Check sheet for the modelled part. Datum: model origin and axes. Units: mm. Face numbers are marked on the shaded views. Coordinates: 2 decimals unless noted, no trailing zeros. Loops run counter-clockwise (first coordinate to the right, second up) from the corner with the lowest first, then second, coordinate; pieces in that order, holes last.
```python
from build123d import *

# Parameters (mm, degrees)
SKETCH013_W     = 47
SKETCH013_H     = 14.8
PAD005_DEPTH    = 3
SKETCH014_R     = 0.95
POCKET003_DEPTH = 5
SKETCH015_R     = 0.95
POCKET004_DEPTH = 2
SKETCH016_W     = 40
SKETCH016_H     = 12.6
PAD006_DEPTH    = 1.5
SKETCH017_R     = 2.5
POCKET005_DEPTH = 10
CHAMFER014_SIZE = 0.5
CHAMFER015_SIZE = 0.5
CHAMFER016_SIZE = 0.2


with BuildPart() as part:
    # Sketch013 → Pad005 (new body)
    with BuildSketch(Plane.YZ):
        with Locations((0, 4.5)):
            Rectangle(SKETCH013_W, SKETCH013_H)
    extrude(amount=PAD005_DEPTH)

    # Sketch014 → Pocket003 (cut)
    with BuildSketch(Plane.YZ):
        with Locations((-21.7, 4.5)):
            Circle(SKETCH014_R)
        with Locations((21.7, 4.5)):
            Circle(SKETCH014_R)
    extrude(amount=POCKET003_DEPTH, mode=Mode.SUBTRACT)

    # Sketch015 → Pocket004 (cut)
    with BuildSketch(Plane.YZ.offset(3)):
        with Locations((-21.7, 4.5)):
            Circle(SKETCH015_R)
        with Locations((21.7, 4.5)):
            Circle(SKETCH015_R)
    extrude(amount=-POCKET004_DEPTH, mode=Mode.SUBTRACT)

    # Sketch016 → Pad006 (join)
    with BuildSketch(Plane.YZ):
        with Locations((0, 4.5)):
            Rectangle(SKETCH016_W, SKETCH016_H)
    extrude(amount=-PAD006_DEPTH)

    # Sketch017 → Pocket005 (cut)
    with BuildSketch(Plane(origin=(3, 15, 4.5), x_dir=(0, 1, 0), z_dir=(1, 0, 0))):
        Circle(SKETCH017_R)
    extrude(amount=-POCKET005_DEPTH, mode=Mode.SUBTRACT)

    # Chamfer014
    chamfer014_edges = [part.edges().sort_by_distance(p)[0] for p in [
        (-1.5, 12.5, 4.5),
        (3, 12.5, 4.5),
    ]]
    chamfer(chamfer014_edges, length=CHAMFER014_SIZE)

    # Chamfer015
    chamfer015_edges = [part.edges().sort_by_distance(p)[0] for p in [
        (-1.5, 20, 4.5),
        (-1.5, 0, -1.8),
        (-1.5, -20, 4.5),
        (-1.5, 0, 10.8),
    ]]
    chamfer(chamfer015_edges, length=CHAMFER015_SIZE)

    # Chamfer016
    chamfer016_edges = [part.edges().sort_by_distance(p)[0] for p in [
        (0, 23.5, 4.5),
        (0, 0, -2.9),
        (0, 0, 11.9),
        (0, -23.5, 4.5),
    ]]
    chamfer(chamfer016_edges, length=CHAMFER016_SIZE)


with BuildPart() as part_1:
    # Body003 placement: moved
    add(part.part.moved(Location((22, 0, 5))))


solid = part_1.part
```
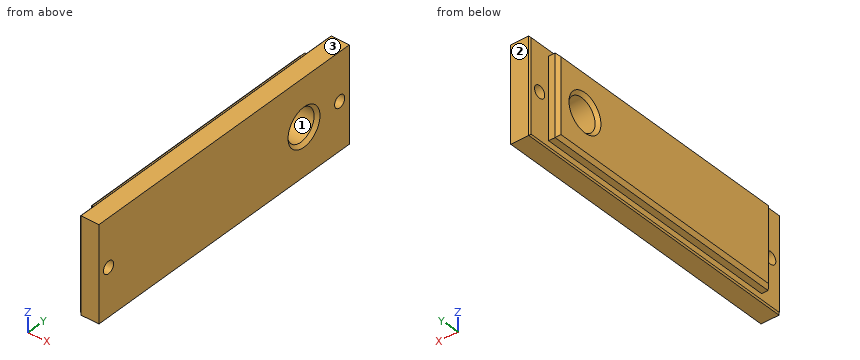
1) Section check D-D on z = 14. Enter the section's corners in (x, y), plus the area to 3 significant figures.
Answer sheet:
outline: (20.5, -19.5) - (21, -20) - (22, -20) - (22, -23.3) - (22.2, -23.5) - (25, -23.5) - (25, 23.5) - (22.2, 23.5) - (22, 23.3) - (22, 20) - (21, 20) - (20.5, 19.5) - close
area: 201 mm2
2) Depth check by flat-ended pin: pin 1 (2.5 mm diameter, centred on y = 21.7, z = 9.5, fed in from +X); pin 2 (0.8 mm diameter, centred on x = 21.5, z = 9.5, fed in from -Y). Enter the tip coordinate at first touch or a pass-through.
Answer sheet:
pin 1: stops at x = 25
pin 2: stops at y = -20
3) Mould release check, pull along Z, two halves, no side actions. Record for the marked faces 1, 2 and 3: +Z half, -Z half, draft (parallel to the pull), parting line (faces both ways), or undercut.
Answer sheet:
face 1: undercut
face 2: draft
face 3: +Z half
4) Scan lines: line 1 (Z direction, x = 22.85, y = -21.7); line 2 (Y direction, x = 24.35, z = 9); line 3 (Z direction, x = 22.6, y = 15). Record each from-to range of solid material in increasing order.
Answer sheet:
line 1: z = 2.1 to 8.55, 10.45 to 16.9
line 2: y = -23.5 to -22.51, -20.89 to 12.55, 17.45 to 20.89, 22.51 to 23.5
line 3: z = 2.1 to 7, 12 to 16.9
5) Section check A-A on z = 9.5. Enter the section's corners in (x, y).
Answer sheet:
outline: (20.5, -19.5) - (21, -20) - (22, -20) - (22, -20.75) - (25, -20.75) - (25, 12) - (24.5, 12.5) - (21, 12.5) - (20.5, 12) - close; (20.5, 18) - (21, 17.5) - (24.5, 17.5) - (25, 18) - (25, 20.75) - (22, 20.75) - (22, 20) - (21, 20) - (20.5, 19.5) - close; (22, -23.3) - (22.2, -23.5) - (25, -23.5) - (25, -22.65) - (22, -22.65) - close; (22, 22.65) - (25, 22.65) - (25, 23.5) - (22.2, 23.5) - (22, 23.3) - close
6) Section check B-B on y = 15. Enter the section's corners in (x, z).
Answer sheet:
outline: (20.5, 3.7) - (21, 3.2) - (22, 3.2) - (22, 2.3) - (22.2, 2.1) - (25, 2.1) - (25, 6.5) - (24.5, 7) - (21, 7) - (20.5, 6.5) - close; (20.5, 12.5) - (21, 12) - (24.5, 12) - (25, 12.5) - (25, 16.9) - (22.2, 16.9) - (22, 16.7) - (22, 15.8) - (21, 15.8) - (20.5, 15.3) - close
7) Section check C-C on x = 23.8. Enter the section's corners in (y, z).
Answer sheet:
outline: (-23.5, 2.1) - (23.5, 2.1) - (23.5, 16.9) - (-23.5, 16.9) - close; hole circle Ø1.9 at (-21.7, 9.5); hole circle Ø5 at (15, 9.5); hole circle Ø1.9 at (21.7, 9.5)
